from build123d import *

# Parameters (mm, degrees)
SKETCH1_W           = 194
SKETCH1_H           = 156
SKETCH1_W_2         = 166
SKETCH1_H_2         = 67
SKETCH1_W_3         = 59
SKETCH1_H_3         = 64
SKETCH1_W_4         = 28
SKETCH1_H_4         = 52
SKETCH1_W_5         = 77
SKETCH1_H_5         = 55
BOSS_EXTRUDE1_DEPTH = 17
SKETCH2_W           = 194
SKETCH2_H           = 156
BOSS_EXTRUDE2_DEPTH = 10
SKETCH3_R           = 2
CUT_EXTRUDE1_DEPTH  = 30


with BuildPart() as part:
    # Sketch1 → Boss-Extrude1 (new body)
    with BuildSketch(Plane(origin=(0, 0, 0), x_dir=(1, 0, 0), z_dir=(0, 1, 0))):
        with Locations((4, 34.5)):
            Rectangle(SKETCH1_W, SKETCH1_H)
        Rectangle(SKETCH1_W_2, SKETCH1_H_2, mode=Mode.SUBTRACT)
        with Locations((-53.5, 70.5)):
            Rectangle(SKETCH1_W_3, SKETCH1_H_3, mode=Mode.SUBTRACT)
        with Locations((-5, 64.5)):
            Rectangle(SKETCH1_W_4, SKETCH1_H_4, mode=Mode.SUBTRACT)
        with Locations((52.5, 66)):
            Rectangle(SKETCH1_W_5, SKETCH1_H_5, mode=Mode.SUBTRACT)
    extrude(amount=BOSS_EXTRUDE1_DEPTH)

    # Sketch2 → Boss-Extrude2 (add)
    with BuildSketch(Plane(origin=(0, 0, 0), x_dir=(-1, 0, 0), z_dir=(0, -1, 0))):
        with Locations((-4, 34.5)):
            Rectangle(SKETCH2_W, SKETCH2_H)
    extrude(amount=BOSS_EXTRUDE2_DEPTH)

    # Sketch3 → Cut-Extrude1 (cut)
    with BuildSketch(Plane(origin=(0, -10, 0), x_dir=(-1, 0, 0), z_dir=(0, -1, 0))):
        with Locations(Location((88, -38.5, 0), (0, 0, 90))):
            Circle(SKETCH3_R)
        with Locations(Location((88, 107.5, 0), (0, 0, 90))):
            Circle(SKETCH3_R)
        with Locations(Location((-96, -38.5, 0), (0, 0, 90))):
            Circle(SKETCH3_R)
        with Locations(Location((-96, 107.5, 0), (0, 0, 90))):
            Circle(SKETCH3_R)
    extrude(amount=-CUT_EXTRUDE1_DEPTH, mode=Mode.SUBTRACT)


solid = part.part
Model file for the job. Use its own axes, mm. A direction names the side the tool comes from. Round coordinates to 2 decimals unless told otherwise and drop trailing zeros. Loops run counter-clockwise (first coordinate to the right, second up) from the corner with the lowest first, then second, coordinate; pieces in that order, holes last.
1. Band-saw the part on A-A, the plane z = -4.5. List the corners of the cut face in (x, y).
Check values:
outline: (-93, -10) - (101, -10) - (101, 17) - (83, 17) - (83, 0) - (-83, 0) - (-83, 17) - (-93, 17) - close
2. Band-saw the part on B-B, the plane y = 11.75. Count the separate pieces of the cut face and the enclosed holes in it, and give its area (3 significant figures).
Check values:
separate pieces: 1
enclosed holes: 8
area: 9,620 mm2
3. Band-saw the part on D-D, the plane x = -11.5. List the corners of the cut face in (y, z).
Check values:
outline: (-10, -112.5) - (17, -112.5) - (17, -90.5) - (0, -90.5) - (0, -38.5) - (17, -38.5) - (17, -33.5) - (0, -33.5) - (0, 33.5) - (17, 33.5) - (17, 43.5) - (-10, 43.5) - close
4. Wall check: probe 1 along Z at (x, y) = (23, 15); probe 2 along X at (y, z) = (0, -107.5); probe 3 along X at (y, z) = (13, -79.5). Give the ranges that are in metal, low to high.
Check values:
probe 1: z = -112.5 to -93.5, -38.5 to -33.5, 33.5 to 43.5
probe 2: x = -93 to -90, -86 to 94, 98 to 101
probe 3: x = -93 to -83, -24 to -19, 9 to 14, 91 to 101
5. Drop a flat-ended pin along its axis: P1, Ø10, axis at x = -44.5, z = 25, coming from the +Y side. Give the stop position or say it passes through.
Check values:
P1: stops at y = 0
6. Tool access for faces 1 (the flat face through (5, -10, -36)), 2 (the flat face through (-53, 0, -71)): list every direction of +Z, -Z, +X, -X, +Y, -Y with a clear straight run to the whole face (end or side of a thin tool).
Check values:
face 1: +Z, -Z, +X, -X, -Y
face 2: +Y
7. Band-saw the part on C-C, the plane x = 76. List the corners of the cut face in (y, z).
Check values:
outline: (-10, -112.5) - (17, -112.5) - (17, -93.5) - (0, -93.5) - (0, -38.5) - (17, -38.5) - (17, -33.5) - (0, -33.5) - (0, 33.5) - (17, 33.5) - (17, 43.5) - (-10, 43.5) - close
8. Mould opens along Z. For faces 3 (the cylindrical face through (-86.017, 3.311, 38.76)), 4 (the flat face through (5, 4, -112.5)), 5 (the flat face through (5, 4, 43.5)) say: +Z half, -Z half, draft (parallel to the pull), parting line (faces both ways), or undercut.
Check values:
face 3: undercut
face 4: -Z half
face 5: +Z half
